The model under review builds one solid part; all positions refer to its coordinate system, in mm. A direction names the side the tool comes from. Give positions to 0.01 mm unless a question says otherwise; leave off trailing zeros. Order: outer loops, then holes, each group sorted by start corner. A loop starts at its lowest first (then second) coordinate and runs counter-clockwise, first axis right, second up. Notation, with made-up numbers: (34, 31.5) -> (38, 31.5) arc R20 cw to (38, 39.5) -> close; hole circle Ø4 at (47.25, -37). An arc over 180 degrees is marked (long way). Use one line per item in the form item = value.
Autodesk Inventor part; units mm, degrees
ref_plane "YZ Plane" through (0, 0, 0) normal (1, 0, 0) x (0, 1, 0)
ref_plane "XZ Plane" through (0, 0, 0) normal (0, 1, 0) x (-1, 0, 0)
ref_plane "XY Plane" through (0, 0, 0) normal (0, 0, 1) x (1, 0, 0)
sketch "Skizze1" plane through (0, 0, 0) normal (1, 0, 0) x (0, 1, 0)
  line L0 (123.2117, 108.1983) -> (122.2117, 109.1983) construction
  line L1 (122.2117, 133.1983) -> (122.2117, 107.1983) construction
  line L2 (122.2117, 107.1983) -> (205.2117, 107.1983) construction
  line L3 (205.2117, 107.1983) -> (205.2117, 133.1983) construction
  line L4 (203.2117, 133.1983) -> (204.2117, 132.1983) construction
  line L5 (122.2117, 107.1983) -> (205.2117, 107.1983)
  line L6 (205.2117, 107.1983) -> (205.2117, 133.1983)
  line L7 (203.2117, 109.1983) -> (123.2703, 109.1983)
  line L8 (123.1703, 108.0983) -> (122.2117, 109.0569)
  line L9 (122.2117, 109.0569) -> (122.2117, 107.1983)
  line L10 (123.2703, 108.0983) -> (123.2703, 109.1983)
  line L11 (123.1703, 108.0983) -> (123.2703, 108.0983)
  line L12 (203.3531, 133.1983) -> (204.3531, 132.1983)
  line L13 (205.2117, 133.1983) -> (203.3531, 133.1983)
  line L14 (204.3531, 132.1983) -> (204.3531, 132.0483)
  line L15 (204.3531, 132.0483) -> (203.2117, 132.0483)
  line L16 (203.2117, 132.0483) -> (203.2117, 109.1983)
  point P0 (0, 0)
  dimension "d2" = 0.1
  dimension "d4" = 2
  dimension "d6" = 1.1
  dimension "d8" = 0.1
  dimension "d9" = 0.1
  dimension "d10" = 0.15
  dimension "d11" = 2
extrude "Extrusion1" add sketch "Skizze1" along normal blind 95
sketch "Skizze2" plane through (0, 0, 0) normal (-1, 0, 0) x (0, 0, 1)
  line L0 (107.1983, 205.2117) -> (133.1983, 205.2117)
  line L1 (109.0569, 122.2117) -> (107.1983, 122.2117)
  line L2 (133.1983, 205.2117) -> (107.1983, 205.2117)
  line L3 (107.1983, 205.2117) -> (107.1983, 122.2117)
  line L4 (107.1983, 122.2117) -> (133.1983, 122.2117)
  line L5 (133.1983, 122.2117) -> (133.1983, 205.2117)
  point P0 (0, 0)
extrude "Extrusion2" add sketch "Skizze2" along normal blind 2.5
properties part number "Batcap2"
1. Add section C-C on z = 127.75. Give the boundary of the cut face in (x, y), then the cut area to 4 significant figures.
Values:
outline = (-2.5, 122.21) -> (0, 122.21) -> (0, 203.21) -> (95, 203.21) -> (95, 205.21) -> (-2.5, 205.21) -> close
area = 397.5 mm^2
2. Tool access review of faces 1 (the face through (95, 176, 109)), 2 (the face through (47, 164, 109.198)): name each direction out of +Z, -Z, +X, -X, +Y, -Y from which nothing blocks a thin tool from reaching the whole face with its end or side.
Values:
face_1 = +Z, -Z, +X, +Y, -Y
face_2 = +Z, +X, -Y
3. For L1, parallel to Z at x = 81.5, y = 146.5; L2, parallel to X at y = 171.5, z = 114.75; L3, parallel to Y at x = 68, z = 116.75, list the stretches that pass through material, from the lowest coordinate up.
Values:
L1 = 107.2 to 109.2
L2 = -2.5 to 0
L3 = 203.21 to 205.21
4. Add section A-A on x = 8. Give the boundary of the cut face in (y, z).
Values:
outline = (122.21, 107.2) -> (205.21, 107.2) -> (205.21, 133.2) -> (203.35, 133.2) -> (204.35, 132.2) -> (204.35, 132.05) -> (203.21, 132.05) -> (203.21, 109.2) -> (123.27, 109.2) -> (123.27, 108.1) -> (123.17, 108.1) -> (122.21, 109.06) -> close
5. Add section B-B on y = 172. Give the boundary of the cut face in (x, z), then the cut area to 3 significant figures.
Values:
outline = (-2.5, 107.2) -> (95, 107.2) -> (95, 109.2) -> (0, 109.2) -> (0, 133.2) -> (-2.5, 133.2) -> close
area = 255 mm^2
6. For pin 1 Ø12 at (x, z) = (50.5, 121.5) entering from -Y; pin 2 Ø8 at (y, z) = (177.5, 125) entering from +X; pin 3 Ø3 at (x, y) = (75.5, 151) entering from +Z, all flat-tipped, find the tip position at first contact; note any pin that passes through.
Values:
pin_1 = 203.21
pin_2 = 0
pin_3 = 109.2
